The drawing under review shows one solid part. Ordinate dimensions are in mm from its lowest x, y, z. A direction names the side the tool comes from. Coordinates: 2 decimals unless noted, no trailing zeros. Loops run counter-clockwise (first coordinate to the right, second up) from the corner with the lowest first, then second, coordinate; pieces in that order, holes last. Notation, with made-up numbers: (26, 55.5) -> (75, 55.5) arc R18 ccw to (75, 74.5) -> close; hole circle Ø6 at (-2.5, -19). An arc over 180 degrees is marked (long way). Use a Markdown table: item, result.
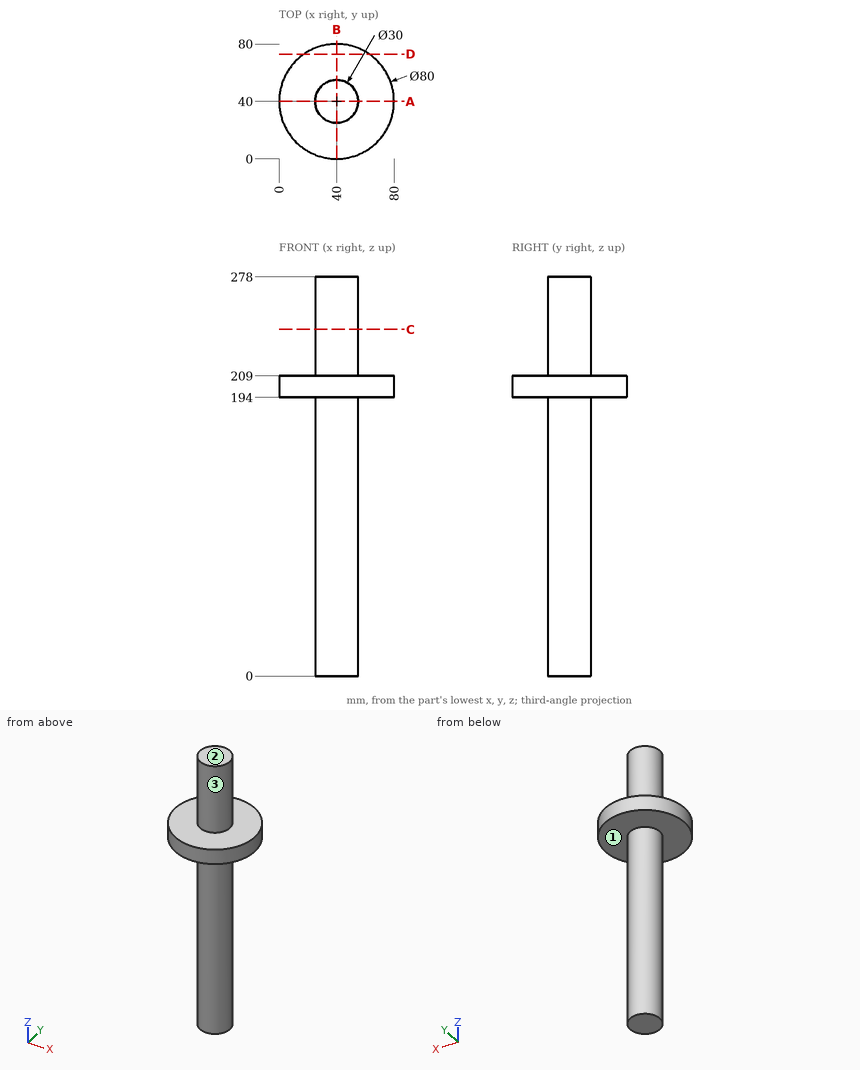
(1) Take a section at A-A on y = 40. Write out the cut boundary in (x, z), plus the area to 3 significant figures.
Found:
| item | result |
|---|---|
| outline | (0, 194) -> (25, 194) -> (25, 0) -> (55, 0) -> (55, 194) -> (80, 194) -> (80, 209) -> (55, 209) -> (55, 278) -> (25, 278) -> (25, 209) -> (0, 209) -> close |
| area | 9,090 mm^2 |
(2) For pin 1 Ø3 at (y, z) = (57.5, 249) entering from +X; pin 2 Ø1 at (x, z) = (35.5, 76.5) entering from +Y; pin 3 Ø2 at (x, z) = (42.5, 136.5) entering from +Y, all flat-tipped, find the tip position at first contact; note any pin that passes through.
Found:
| item | result |
|---|---|
| pin 1 | passes through |
| pin 2 | stops at y = 54.46 |
| pin 3 | stops at y = 54.92 |
(3) Take a section at D-D on y = 73. Write out the cut boundary in (x, z), plus the area to 3 significant figures.
Found:
| item | result |
|---|---|
| outline | (17.39, 194) -> (62.61, 194) -> (62.61, 209) -> (17.39, 209) -> close |
| area | 678 mm^2 |
(4) For the marked faces 1, 2 and 3, list the 3-axis set-ups (+Z, -Z, +X, -X, +Y, -Y) from which the entire face can be reached by the end or side of a thin tool; tool diameter is ignored.
Found:
| item | result |
|---|---|
| face 1 | -Z |
| face 2 | +Z, +X, -X, +Y, -Y |
| face 3 | +Z |
(5) Take a section at C-C on z = 241.5. Write out the cut boundary in (x, y), plus the area to 3 significant figures.
Found:
| item | result |
|---|---|
| outline | circle Ø30 at (40, 40) |
| area | 707 mm^2 |
(6) For line 1 along Z through (x, y) = (38.5, 76); line 2 along Y through (x, z) = (40.5, 87); line 3 along Y through (x, z) = (53, 36.5), list the stretches that pass through material, from the lowest coordinate up.
Found:
| item | result |
|---|---|
| line 1 | z = 194 to 209 |
| line 2 | y = 25.01 to 54.99 |
| line 3 | y = 32.52 to 47.48 |
